For this review, take the finished solid that the model builds, in its own axes (mm). A direction names the side the tool comes from. Round coordinates to 2 decimals unless told otherwise and drop trailing zeros. Write each loop counter-clockwise with the first axis right and the second up, starting at its lowest first coordinate (ties: lowest second). Pieces come first, ordered by that corner, then holes. Notation, with made-up numbers: (65.5, 54) - (103.5, 54) arc R22 ccw to (103.5, 67) - close; hole circle Ø1 at (11, -18.5). An arc over 180 degrees is marked (long way). One line per item, written item: value. Start each with the question number.
Q1. Add section C-C on z = -8. Write out the cut boundary in (x, y), and give its area (3 significant figures).
Q2. Mouldability with a two-part tool opening along Z and no side actions: class faces 4 (the face through (-25.23, 0.49, -12.22)), 5 (the face through (-21.772, 0.493, 21.976)), 6 (the face through (-22.5, 0.5, 30.828)), 7 (the face through (12.202, 0.5, -7.6)) as +Z half, -Z half, draft (parallel to the pull), parting line (faces both ways), or undercut.
Q3. Add section A-A on x = 10.5. Write out the cut boundary in (y, z).
Q4. Clearance check with flat-ended pins moving along their axes: pin 1 Ø2.5 at (x, z) = (4.7, 23.33) entering from +Y; pin 2 Ø6.5 at (x, z) = (9.2, -14.17) entering from +Y. State where each tip first meets the part, or that it passes through.
Q5. Add section B-B on y = 0.65. Write out the cut boundary in (x, z), and give its area (3 significant figures).
Q6. Tool access review of faces 1 (the face through (-27.798, 0.5, 25.3)), 2 (the face through (-27.798, 0.5, -7.9)), 3 (the face through (12.202, 0.5, 25.5)): name each direction out of +Z, -Z, +X, -X, +Y, -Y from which nothing blocks a thin tool from reaching the whole face with its end or side.
Q7. For probe 1 along X at (y, z) = (0.4, -13.5); probe 2 along X at (y, z) = (0.8, -2.5); probe 3 along Z at (x, y) = (-8, 0.3), list the stretches that pass through material, from the lowest coordinate up.
Q8. Add section D-D on x = -14.5. Write out the cut boundary in (y, z), and give its area (3 significant figures).
```python
from build123d import *

# Parameters (mm, degrees)
SKETCH1_R           = 2
BOSS_EXTRUDE1_DEPTH = 1


with BuildPart() as part:
    # Sketch1 → Boss-Extrude1 (new body)
    with BuildSketch(Plane(origin=(0, 0, 0), x_dir=(1, 0, 0), z_dir=(0, 1, 0))):
        with BuildLine():
            Line((12.20211229, -1.662478542), (12.20211229, 17.172370068))
            Line((12.20211229, 17.172370068), (-27.79788771, 17.172370068))
            Line((-27.79788771, 17.172370068), (-27.79788771, -1.662478542))
            ThreePointArc((-27.79788771, -1.662478542), (-29.79788771, -10.827629932), (-27.79788771, -19.992781322))
            Line((-27.79788771, -19.992781322), (-27.79788771, -30.827629932))
            Line((-27.79788771, -30.827629932), (-16.9630391, -30.827629932))
            ThreePointArc((-16.9630391, -30.827629932), (-7.79788771, -32.827629932), (1.36726368, -30.827629932))
            Line((1.36726368, -30.827629932), (12.20211229, -30.827629932))
            Line((12.20211229, -30.827629932), (12.20211229, -19.992781322))
            ThreePointArc((12.20211229, -19.992781322), (14.20211229, -10.827629932), (12.20211229, -1.662478542))
        make_face()
        with Locations((-20.29788771, -23.327629932)):
            Circle(SKETCH1_R, mode=Mode.SUBTRACT)
        with Locations((4.70211229, -23.327629932)):
            Circle(SKETCH1_R, mode=Mode.SUBTRACT)
        with Locations((-24.79788771, 14.172370068)):
            Circle(SKETCH1_R, mode=Mode.SUBTRACT)
        with Locations((9.20211229, 14.172370068)):
            Circle(SKETCH1_R, mode=Mode.SUBTRACT)
    extrude(amount=BOSS_EXTRUDE1_DEPTH)


solid = part.part
```
Result set:
1. outline: (-27.8, 0) - (12.2, 0) - (12.2, 1) - (-27.8, 1) - close
1. area: 40.0 mm^2
2. face 4: undercut
2. face 5: undercut
2. face 6: +Z half
2. face 7: draft
3. outline: (0, -17.17) - (1, -17.17) - (1, -15.69) - (0, -15.69) - close; (0, -12.65) - (1, -12.65) - (1, 30.83) - (0, 30.83) - close
4. pin 1: passes through
4. pin 2: stops at y = 1
5. outline: (-27.8, -17.17) - (12.2, -17.17) - (12.2, 1.66) arc R22 ccw to (12.2, 19.99) - (12.2, 30.83) - (1.37, 30.83) arc R22 ccw to (-16.96, 30.83) - (-27.8, 30.83) - (-27.8, 19.99) arc R22 ccw to (-27.8, 1.66) - close; hole circle Ø4 at (-24.8, -14.17); hole circle Ø4 at (-20.3, 23.33); hole circle Ø4 at (4.7, 23.33); hole circle Ø4 at (9.2, -14.17)
5. area: 1,940 mm^2
6. face 1: +Z, -X, +Y, -Y
6. face 2: -Z, -X, +Y, -Y
6. face 3: +Z, +X, +Y, -Y
7. probe 1: x = -27.8 to -26.68, -22.91 to 7.32, 11.09 to 12.2
7. probe 2: x = -27.8 to 12.2
7. probe 3: z = -17.17 to 32.83
8. outline: (0, -17.17) - (1, -17.17) - (1, 31.78) - (0, 31.78) - close
8. area: 49.0 mm^2
